CAD build for the part. Positions are in the model's coordinates, mm. A direction names the side the tool comes from. Give positions to 0.01 mm unless a question says otherwise; leave off trailing zeros. Write each loop counter-clockwise with the first axis right and the second up, starting at its lowest first coordinate (ties: lowest second). Pieces come first, ordered by that corner, then holes. Notation, with made-up numbers: (-30.75, 45) - (-20.75, 45) arc R4 cw to (-20.75, 50) - close; hole circle Ø11 at (-31, 14.25). An arc over 180 degrees is marked (long way). Answer as a JSON object with one key per item and string values.
from build123d import *

# Parameters (mm, degrees)
BASE_FLANGE1_DEPTH  = 2.5
SKETCH6_W           = 0.4
SKETCH6_H           = 3.67
BOSS_EXTRUDE1_DEPTH = 4.5
SKETCH7_W           = 3.4
SKETCH7_H           = 1
CUT_EXTRUDE1_DEPTH  = 12.139958989
FILLET1_RADIUS      = 1.335
FILLET1_LENGTH      = 0.4
SCALE1_SCALE        = 10


# Sheet-metal steps are written as plain solids
with BuildPart() as part:
    # Sketch1 → Base-Flange1 (new body)
    with BuildSketch(Plane.XY):
        with BuildLine():
            Line((0.71, -1.835), (0.71, 1.835))
            ThreePointArc((0.71, 1.835), (0, 2.545), (-0.71, 1.835))
            Line((-0.71, 1.835), (-0.71, -2.335))
            ThreePointArc((-0.71, -2.335), (-1.228475759, -3.211432773), (-2.246268811, -3.179047252))
            Line((-2.246268811, -3.179047252), (-6.888528694, -0.229568793))
            Line((-6.888528694, -0.229568793), (-6.67402117, 0.108050107))
            Line((-6.67402117, 0.108050107), (-2.031761286, -2.841428351))
            ThreePointArc((-2.031761286, -2.841428351), (-1.421085455, -2.860859664), (-1.11, -2.335))
            Line((-1.11, -2.335), (-1.11, 1.835))
            ThreePointArc((-1.11, 1.835), (0, 2.945), (1.11, 1.835))
            Line((1.11, 1.835), (1.11, -1.835))
            Line((1.11, -1.835), (0.71, -1.835))
        make_face()
    extrude(amount=BASE_FLANGE1_DEPTH)

    # Sketch6 → Boss-Extrude1 (add)
    with BuildSketch(Plane.XY.offset(2.5)):
        with Locations((0.91, 0)):
            Rectangle(SKETCH6_W, SKETCH6_H)
    extrude(amount=BOSS_EXTRUDE1_DEPTH)

    # Sketch7 → Cut-Extrude1 (cut, through all)
    with BuildSketch(Plane(origin=(1.11, 0, 0), x_dir=(0, 0, -1), z_dir=(1, 0, 0))):
        with Locations((-5.3, -1.335)):
            Rectangle(SKETCH7_W, SKETCH7_H)
    extrude(amount=-CUT_EXTRUDE1_DEPTH, mode=Mode.SUBTRACT)

    # Fillet1: full round fillet: the end face becomes a half cylinder, R = half its width
    fillet1_face = Plane((0.91, 0.5, 7), x_dir=(-1, 0, 0), z_dir=(0, 0, 1))  # on the end face: x along it, z out of the body
    fillet1_slab = fillet1_face.offset(-FILLET1_RADIUS / 2) * Box(FILLET1_LENGTH, 2 * FILLET1_RADIUS, FILLET1_RADIUS, mode=Mode.PRIVATE)  # the body's end, R deep
    fillet1_round = Plane((0.91, 0.5, 5.665), x_dir=(0, 0, 1), z_dir=(-1, 0, 0)) * Cylinder(FILLET1_RADIUS, FILLET1_LENGTH, mode=Mode.PRIVATE)  # its axis R under the face
    add(fillet1_slab - fillet1_round, mode=Mode.SUBTRACT)


with BuildPart() as part_1:
    # Scale1: scaled about (-1.000602335, -0.257853748, 1.947858074)
    add(part.part.scale(SCALE1_SCALE).moved(Location((9.005421015, 2.320683732, -17.530722666))))


solid = part_1.part
(1) Flat gauge pins, fed straight in: P1, Ø2, axis at x = 18, y = -9, coming from the +Z side; P2, Ø3, axis at x = 18.5, z = 34, coming from the -Y side; P3, Ø1.5, axis at y = -5.5, z = 34.5, coming from the -X side. Where does each tip first touch, or does it go through?
Answer key:
{"P1": "stops at z = 18.47", "P2": "stops at y = -6.03", "P3": "stops at x = 16.11"}
(2) Saw through at B-B, the plane z = -12.5. Give the cut face in (x, y) (3 decimals), and give its area (3 significant figures).
Answer key:
{"outline": "(-59.88, 0.025) - (-13.457, -29.47) arc R10 ccw to (1.905, -21.029) - (1.905, 20.671) arc R7.1 cw to (16.105, 20.671) - (16.105, -16.029) - (20.105, -16.029) - (20.105, 20.671) arc R11.1 ccw to (-2.095, 20.671) - (-2.095, -21.029) arc R6 cw to (-11.312, -26.094) - (-57.735, 3.401) - close", "area": "716 mm²"}
(3) Saw through at A-A, the plane y = -1.5. Give the cut face in (x, z).
Answer key:
{"outline": "(-57.48, -17.53) - (-50.02, -17.53) - (-50.02, 7.47) - (-57.48, 7.47) - close; (-2.09, -17.53) - (1.91, -17.53) - (1.91, 7.47) - (-2.09, 7.47) - close; (16.11, -17.53) - (20.11, -17.53) - (20.11, 49.14) - (16.11, 49.14) - close"}
(4) 3-axis set-ups, long thin cutter, end or side, ignore diameter. For faces 1 (the face through (18, -16.029, 0)), 2 (the face through (-2.095, 0, -5)), 3 (the face through (16.105, 2, 9)), 4 (the face through (18, -6.029, 29)), 5 (the face through (18, 20.671, 23)): which of +Z, -Z, +X, -X, +Y, -Y reach the whole face in a straight line?
Answer key:
{"face 1": "+Z, -Z, +X, -Y", "face 2": "+Z, -Z, +Y", "face 3": "+Z, -Z, -Y", "face 4": "+Z, +X, -X, -Y", "face 5": "+Z, +X, -X, +Y"}
(5) Probe L1, parallel to X at y = 6, z = -4; L2, parallel to X at y = 3, z = 40; L3, parallel to X at y = -6.5, z = -10. List the from-to ranges inside material, lowest first. Write a range as [from, to].
Answer key:
{"L1": "x = [-2.09, 1.91], [16.11, 20.11]", "L2": "x = [16.11, 20.11]", "L3": "x = [-49.61, -42.15], [-2.09, 1.91], [16.11, 20.11]"}
(6) Saw through at C-C, the plane y = 17.5. Give the cut face in (x, z), and give its area (3 significant figures).
Answer key:
{"outline": "(-2.09, -17.53) - (1.91, -17.53) - (1.91, 7.47) - (-2.09, 7.47) - close; (16.11, -17.53) - (20.11, -17.53) - (20.11, 47.76) - (16.11, 47.76) - close", "area": "361 mm²"}
(7) Saw through at D-D, the plane y = -8. Give the cut face in (x, z), and give its area (3 significant figures).
Answer key:
{"outline": "(-47.25, -17.53) - (-39.79, -17.53) - (-39.79, 7.47) - (-47.25, 7.47) - close; (-2.09, -17.53) - (1.91, -17.53) - (1.91, 7.47) - (-2.09, 7.47) - close; (16.11, -17.53) - (20.11, -17.53) - (20.11, 18.47) - (16.11, 18.47) - close", "area": "430 mm²"}
(8) Pull direction X, two halves, no side cores. Call faces 6 (the face through (-34.85, -11.14, -5.21)), 7 (the face through (-3.15, -29.72, -5.21)), 8 (the face through (-1.9, -1.8, -17.531)): pulls with the +X half, pulls with the -X half, needs draft (parallel to the pull), parting line crosses it, or undercut.
Answer key:
{"face 6": "undercut", "face 7": "parting line crosses it", "face 8": "needs draft"}
